Read the model definition and answer for the solid it produces. Units are mm, in the model's axes. A direction names the side the tool comes from. Give positions to 0.01 mm unless a question says otherwise; leave off trailing zeros. Write each loop counter-clockwise with the first axis right and the second up, starting at its lowest first coordinate (ties: lowest second). Pieces come first, ordered by that corner, then holes. Notation, with made-up numbers: (88, -36.5) - (126, -36.5) arc R21 cw to (126, -31.5) - close; hole circle Ø11 at (-8.5, -4). An arc over 180 degrees is marked (long way). Use CSV: the item, a comma, the result in double quotes. Start each with the question number.
from build123d import *

# Parameters (mm, degrees)
SKETCH_R  = 3.3
PAD_DEPTH = 68


with BuildPart() as part:
    # Sketch → Pad (new body)
    with BuildSketch(Plane.XY):
        with BuildLine():
            Line((17, 1.5), (0, 1.5))
            Line((0, 1.5), (0, 0))
            Line((0, 0), (34, 0))
            Line((34, 0), (34, 7.499986))
            ThreePointArc((34, 7.499986), (27.000014, 14.5), (20, 7.500014))
            Line((20, 2.5), (20, 7.500014))
            Line((17, 2.5), (20, 2.5))
            Line((17, 1.5), (17, 2.5))
        make_face()
        with Locations((27, 7.5)):
            Circle(SKETCH_R, mode=Mode.SUBTRACT)
    extrude(amount=PAD_DEPTH)


solid = part.part
(1) For a pull along Y with two mould halves and no side action, classify faces 1 (the face through (9, 1.5, 34)), 2 (the face through (30.05, 6.24, 33.52)), 3 (the face through (34, 4, 34)) as pulls with the +Y half, pulls with the -Y half, needs draft (parallel to the pull), parting line crosses it, or undercut.
(2) The part is cut by section A-A on x = 27. Write down the section's boundary in (y, z).
(3) The part is cut by section B-B on z = 31.5. Write down the section's boundary in (x, y), plus the area to 3 significant figures.
(4) The part is cut by section D-D on x = 18.5. Write down the section's boundary in (y, z), plus the area to 3 significant figures.
(5) Given P1, Ø1, axis at x = 17.5, z = 43.5, coming from the +Y side; P2, Ø2.5, axis at y = 6, z = 39, coming from the -X side; P3, Ø2, axis at x = 10, z = 36, coming from the +Y side, each flat-ended and moving along its own axis, determine where each tip first touches the part or whether it passes through.
(6) Which of the six approach directions +Z, -Z, +X, -X, +Y, -Y give full straight-line access (tool end or side, diameter ignored) to faces 4 (the face through (24, 4, 68)), 5 (the face through (20, 5, 34))?
(7) Consider probe 1 along Y at (x, z) = (27, 33); probe 2 along X at (y, z) = (7.25, 41); probe 3 along Y at (x, z) = (12.5, 47.5). Determine where each line is inside the solid, lowest interval first.
(8) The part is cut by section C-C on y = 8.75. Write down the section's boundary in (x, z), plus the area to 3 significant figures.
Reported:
1,face 1,"pulls with the +Y half"
1,face 2,"undercut"
1,face 3,"needs draft"
2,outline,"(0, 0) - (4.2, 0) - (4.2, 68) - (0, 68) - close; (10.8, 0) - (14.5, 0) - (14.5, 68) - (10.8, 68) - close"
3,outline,"(0, 0) - (34, 0) - (34, 7.5) arc R7 ccw to (20, 7.5) - (20, 2.5) - (17, 2.5) - (17, 1.5) - (0, 1.5) - close; hole circle Ø6.6 at (27, 7.5)"
3,area,"181 mm²"
4,outline,"(0, 0) - (2.5, 0) - (2.5, 68) - (0, 68) - close"
4,area,"170 mm²"
5,P1,"y = 2.5"
5,P2,"x = 20"
5,P3,"y = 1.5"
6,face 4,"+Z, +X, -X, +Y, -Y"
6,face 5,"+Z, -Z, -X, +Y"
7,probe 1,"0 to 4.2, 10.8 to 14.5"
7,probe 2,"20 to 23.71, 30.29 to 34"
7,probe 3,"0 to 1.5"
8,outline,"(20.11, 0) - (23.95, 0) - (23.95, 68) - (20.11, 68) - close; (30.05, 0) - (33.89, 0) - (33.89, 68) - (30.05, 68) - close"
8,area,"521 mm²"
